Study the drawing (mm; zero at the part's minimum x, y, z) and answer. A direction names the side the tool comes from. Coordinates: 2 decimals unless noted, no trailing zeros. Loops run counter-clockwise (first coordinate to the right, second up) from the corner with the lowest first, then second, coordinate; pieces in that order, holes last. Notation, with made-up numbers: (-0.75, 29) -> (8.25, 29) arc R33 ccw to (8.25, 59) -> close; hole circle Ø8 at (10.5, 80.25). An arc over 180 degrees is marked (long way). Answer as CSV lines item,"result".
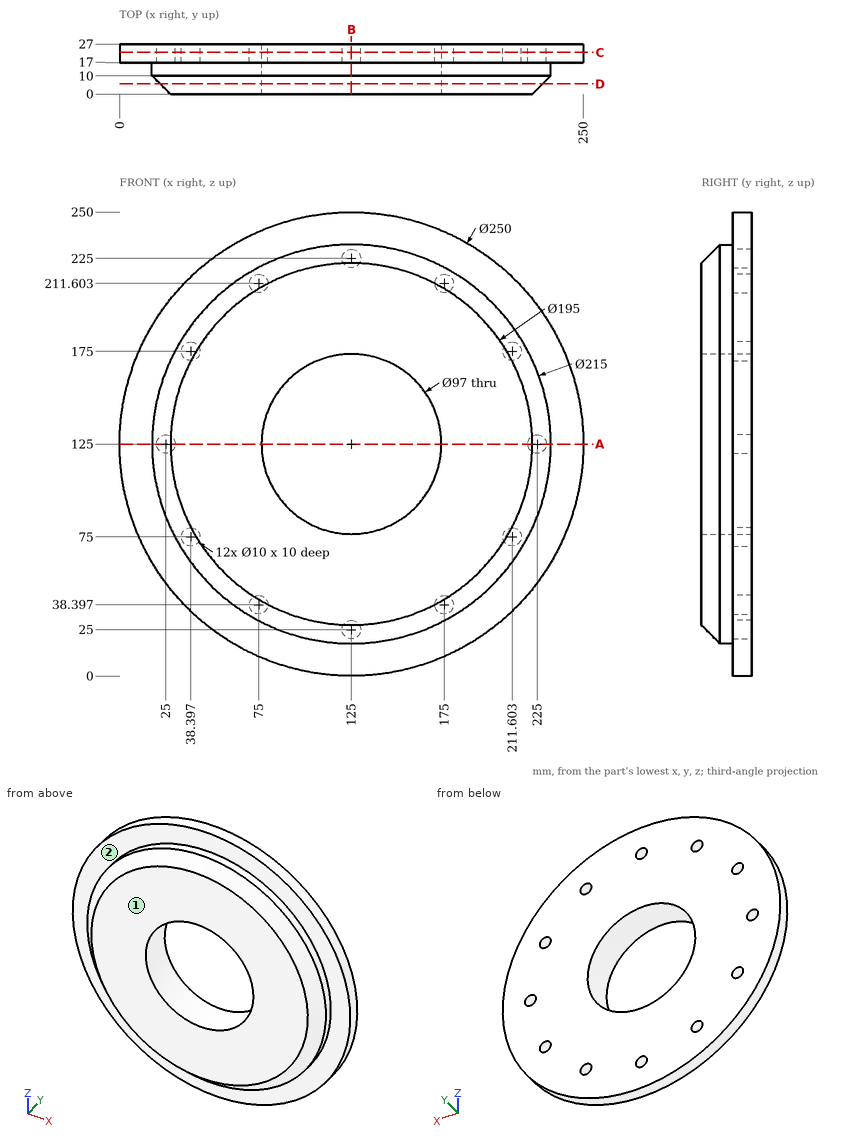
Q1. A cutting plane is placed at D-D, the plane y = 5.5. Write down the section's boundary in (x, z), and give its area (3 significant figures).
Results:
outline,"circle Ø206 at (125, 125); hole circle Ø97 at (125, 125)"
area,"25,900 mm²"
Q2. A cutting plane is placed at C-C, the plane y = 22.5. Give the number of separate pieces and of enclosed holes in the cut face, and give its area (3 significant figures).
Results:
separate pieces,"1"
enclosed holes,"13"
area,"40,800 mm²"
Q3. A cutting plane is placed at A-A, the plane z = 125. Write down the section's boundary in (x, y).
Results:
outline,"(0, 17) -> (17.5, 17) -> (17.5, 10) -> (27.5, 0) -> (76.5, 0) -> (76.5, 27) -> (30, 27) -> (30, 17) -> (20, 17) -> (20, 27) -> (0, 27) -> close; (173.5, 0) -> (222.5, 0) -> (232.5, 10) -> (232.5, 17) -> (250, 17) -> (250, 27) -> (230, 27) -> (230, 17) -> (220, 17) -> (220, 27) -> (173.5, 27) -> close"
Q4. Find the intervals of material crossed by probe 1 along Z at (x, y) = (129.5, 17.5) (1 decimal); probe 2 along Z at (x, y) = (175, 22.25) (1 decimal); probe 3 along Y at (x, z) = (163, 239), in increasing order. Write a range as [from, to].
Results:
probe 1,"z = [0.1, 22.8], [27.2, 76.7], [173.3, 222.8], [227.2, 249.9]"
probe 2,"z = [10.4, 33.4], [43.4, 206.6], [216.6, 239.6]"
probe 3,"y = [17, 27]"
Q5. For the marked faces 1 and 2, determine the directions among +Z, -Z, +X, -X, +Y, -Y from which every point of the face is accessible in a straight line to the end or side of a thin tool.
Results:
face 1,"+Z, -Z, +X, -X, -Y"
face 2,"-Y"
Q6. A cutting plane is placed at B-B, the plane x = 125. Write down the section's boundary in (y, z).
Results:
outline,"(0, 27.5) -> (10, 17.5) -> (17, 17.5) -> (17, 0) -> (27, 0) -> (27, 20) -> (17, 20) -> (17, 30) -> (27, 30) -> (27, 76.5) -> (0, 76.5) -> close; (0, 173.5) -> (27, 173.5) -> (27, 220) -> (17, 220) -> (17, 230) -> (27, 230) -> (27, 250) -> (17, 250) -> (17, 232.5) -> (10, 232.5) -> (0, 222.5) -> close"
Q7. Given pin 1 Ø9 at (x, z) = (38.4, 75) entering from +Y; pin 2 Ø3 at (x, z) = (35, 55.5) entering from -Y; pin 3 Ø1.5 at (x, y) = (37, 14) entering from +Z, each flat-ended and moving along its own axis, determine where each tip first touches the part or whether it passes through.
Results:
pin 1,"stops at y = 17"
pin 2,"stops at y = 17"
pin 3,"stops at z = 187.8"
